```python
from build123d import *

# Parameters (mm, degrees)
EXTRUDE_5_REACH      = 191.138
EXTRUDE_5_END_RADIUS = 48
EXTRUDE_START        = 106
SKETCH_6_R           = 18.746212634
EXTRUDE_5_START      = 106
EXTRUDE_5_DRAFT      = -6
SHELL_2_T            = -2
SKETCH_7_R           = 25
SKETCH_7_R_2         = 16.735196074
EXTRUDE_6_DEPTH      = 5


with BuildPart() as part:
    # Sketch 5 → Revolve 8 (revolve)
    with BuildSketch(Plane.XY):
        with BuildLine():
            Line((0, 48), (0, -48))
            ThreePointArc((0, -48), (48, 0), (0, 48))
        make_face()
    revolve(axis=Axis((0, 48, 0), (0, -1, 0)))

    # Extrude 5: up to this sphere (the profile starts outside it)
    extrude_5_end = Location((0, 0, 0)) * Sphere(EXTRUDE_5_END_RADIUS, mode=Mode.PRIVATE)



with BuildPart() as extrude_5_long_prism_1:
    # Sketch 6 → Extrude 5 (the long prism of profile 1, to be tilted and cut off)
    with BuildSketch(Plane(origin=(0, 0, 0), x_dir=(1, 0, 0), z_dir=(0, 1, 0)).offset(EXTRUDE_START)):
        with Locations((-36.793445322, 0)):
            Circle(SKETCH_6_R)
    extrude(amount=-EXTRUDE_5_REACH)
    extrude_5_tool1_sides = [extrude_5_long_prism_1.faces().sort_by_distance(p)[0] for p in [
        (-55.539657956, 10.431, 0),
    ]]
    draft(extrude_5_tool1_sides, Plane(origin=(0, 0, 0), x_dir=(1, 0, 0), z_dir=(0, 1, 0)).offset(EXTRUDE_5_START), EXTRUDE_5_DRAFT)  # the draft: side faces tilted about the start plane


with BuildPart() as part_1:
    add(part.part)
    extrude_5_tool1 = extrude_5_long_prism_1.part - extrude_5_end
    add(extrude_5_tool1.solids().sort_by_distance((-36.793445, 106, 0))[0])

    # Shell 2
    shell_2_openings = [part_1.faces().sort_by_distance(p)[0] for p in [
        (-36.793445322, 106, 0),
    ]]
    offset(amount=SHELL_2_T, openings=shell_2_openings, kind=Kind.INTERSECTION)

    # Sketch 7 → Extrude 6 (add)
    with BuildSketch(Plane(origin=(0, 106, 0), x_dir=(1, 0, 0), z_dir=(0, 1, 0))):
        with Locations(Location((-36.793445322, 0, 0), (0, 0, 270))):
            Circle(SKETCH_7_R)
        with Locations((-36.793445322, 0)):
            Circle(SKETCH_7_R_2, mode=Mode.SUBTRACT)
    extrude(amount=-EXTRUDE_6_DEPTH)


solid = part_1.part
```
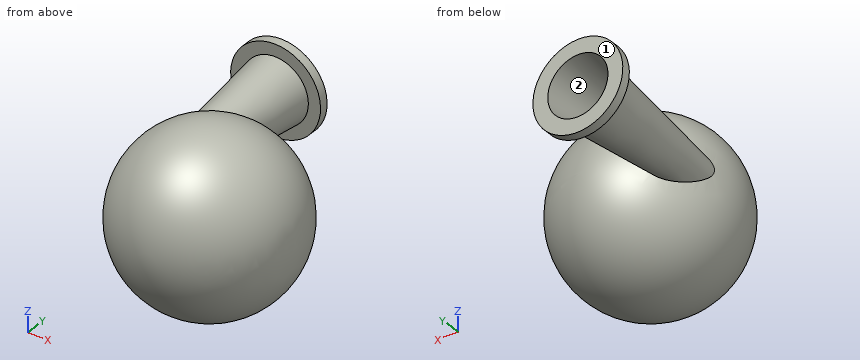
The model under review builds one solid part; all positions refer to its coordinate system, in mm. Face numbers are marked on the shaded views. Round coordinates to 2 decimals unless told otherwise and drop trailing zeros. Loops run counter-clockwise (first coordinate to the right, second up) from the corner with the lowest first, then second, coordinate; pieces in that order, holes last. Notation, with made-up numbers: (0.5, -31.5) - (31.5, -31.5) arc R28 ccw to (31.5, 2.5) - close; hole circle Ø4 at (15, 21). An arc over 180 degrees is marked (long way). Write each question's results on one line, items separated by ' | '. Start each with the question number.
Q1. Take a section at C-C on y = -11.5. Give the boundary of the cut face in (x, z).
Q2. Wall thickness on line 1 along X through (y, z) = (40, -16); line 2 along X through (y, z) = (91.5, 4); line 3 along Y through (x, z) = (3.5, -38.5): over which ranges is each line inside the solid? List them lowest first. Write a range as [from, to].
Q3. Take a section at A-A on x = 12.5. Give the boundary of the cut face in (y, z).
Q4. Draft analysis for pull direction X (two halves, no side actions). For the marked faces 1 and 2, state which applies: pulls with the +X half, pulls with the -X half, needs draft (parallel to the pull), parting line crosses it, or undercut.
Q5. Take a section at B-B on z = 0. Give the boundary of the cut face in (x, y), plus the area to 3 significant figures.
Q6. Insertion check: P1, Ø4, axis at x = 0.5, z = 8.5, coming from the +Y side; P2, Ø1.5, axis at y = 7, z = -1.5, coming from the -X side; P3, Ø8, axis at x = 16, z = -38, coming from the -Y side. Each pin has a flat end and moves straight along its axis. Give the tip position at first contact, or say it passes through.
Data:
1) outline: circle Ø93.2 at (0, 0); hole circle Ø89.08 at (0, 0)
2) line 1: x = [-21.17, -16.12], [16.12, 21.17] | line 2: x = [-53.54, -51.47], [-22.12, -20.04] | line 3: y = [-28.45, -24.93], [24.93, 28.45]
3) outline: circle Ø92.69 at (0, 0); hole circle Ø88.54 at (0, 0)
4) face 1: needs draft | face 2: undercut
5) outline: (-61.79, 101) - (-55.01, 101) - (-45.88, 14.1) arc R48 ccw (long way) to (-24.87, 41.05) - (-18.57, 101) - (-11.79, 101) - (-11.79, 106) - (-20.06, 106) - (-27.31, 37.02) arc R46 cw (long way) to (-43.85, 13.9) - (-53.53, 106) - (-61.79, 106) - close | area: 911 mm²
6) P1: stops at y = 47.56 | P2: stops at x = -47.57 | P3: stops at y = -30.3
